Read the model definition and answer for the solid it produces. Units are mm, in the model's axes. Face numbers are marked on the shaded views. A direction names the side the tool comes from. Round coordinates to 2 decimals unless told otherwise and drop trailing zeros. Write each loop counter-clockwise with the first axis right and the second up, starting at its lowest first coordinate (ties: lowest second). Pieces come first, ordered by that corner, then holes. Notation, with made-up numbers: (-3, 42.25) - (5, 42.25) arc R25 cw to (5, 74.25) - close; hole circle Ø4 at (67.5, 42.25). An arc over 180 degrees is marked (long way). Answer as CSV lines item,"result". Start each with the question number.
1) For a pull along X with two mould halves and no side action, classify the marked faces 1, 2 and 3 as +X half, -X half, draft (parallel to the pull), parting line (faces both ways), or undercut.
2) Consider line 1 along Z through (x, y) = (12.7, 4.5); line 2 along X through (y, z) = (18.5, 19) (3 decimals); line 3 along Z through (x, y) = (-12.7, 2.25). Determine where each line is inside the solid, lowest interval first.
3) Find section D-D on y = 5.5. Determine the outline of the cut face in (x, z) (1 decimal), then the cut area to 3 significant figures.
4) Find section C-C on x = -12.7. Determine the outline of the cut face in (y, z).
5) Find section B-B on z = 34. Determine the outline of the cut face in (x, y) (3 decimals), then the cut area to 3 significant figures.
6) Which of the six approach directions +Z, -Z, +X, -X, +Y, -Y give full straight-line access (tool end or side, diameter ignored) to the marked faces 4, 5 and 6?
7) Find section A-A on y = 20.5. Determine the outline of the cut face in (x, z) (1 decimal), then the cut area to 3 significant figures.
8) Each of these flat-tipped pins is pushed along its axis until it touches: pin 1 (0.5 mm diameter, centred on x = 4, z = -0.5, fed in from +Y); pin 2 (4 mm diameter, centred on x = 12, y = 20, fed in from -Z); pin 3 (1 mm diameter, centred on x = 0, y = 9.5, fed in from +Z); pin 4 (8 mm diameter, centred on x = 4.5, y = 26.5, fed in from -Z). Where does it stop, or does it pass through?
Autodesk Inventor part; units mm, degrees
ref_plane "YZ Plane" through (0, 0, 0) normal (1, 0, 0) x (0, 1, 0)
ref_plane "XZ Plane" through (0, 0, 0) normal (0, 1, 0) x (-1, 0, 0)
ref_plane "XY Plane" through (0, 0, 0) normal (0, 0, 1) x (1, 0, 0)
sketch "Sketch1" plane through (0, 0, 0) normal (0, 0, 1) x (1, 0, 0)
  line L0 (-15.875, 0) -> (15.875, 0)
  line L1 (15.875, 0) -> (15.875, 38.1)
  line L2 (15.875, 38.1) -> (-15.875, 38.1)
  line L3 (-15.875, 38.1) -> (-15.875, 0)
  point P0 (0, 0)
  dimension "d2" = 31.75
  dimension "d3" = 38.1
  dimension "d4" = 15.875
  dimension "d5" = 0
extrude "Extrusion1" add sketch "Sketch1" along normal blind 139.7
sketch "Sketch2" plane through (0, 0, 139.7) normal (0, 0, 1) x (1, 0, 0)
  arc A0 (-12.065, 19.05) -> (12.065, 19.05) centre (0, 19.05) ccw
  line L0 (-15.875, 0) -> (15.875, 0)
  line L1 (12.065, 19.05) -> (12.065, 38.1)
  line L2 (15.875, 38.1) -> (-15.875, 38.1)
  line L3 (-12.065, 19.05) -> (-12.065, 38.1)
  point P0 (0, 0)
  dimension "d8" = 19.05
  dimension "d9" = 24.13
extrude "Extrusion2" cut sketch "Sketch2" against normal through all
sketch "Sketch3" plane through (-15.875, 0, 0) normal (0, -1, 0) x (1, 0, 0)
  circle A0 centre (28.575, 8.89) radius 2
  circle A1 centre (3.175, 130.81) radius 2
  line L0 (15.875, 0) -> (15.875, 139.7) construction
  line L1 (0, 139.7) -> (31.75, 139.7) construction
  line L2 (0, 0) -> (31.75, 0) construction
  line L3 (31.75, 139.7) -> (0, 139.7) construction
  circle A2 centre (3.175, 27.94) radius 2
  dimension "d12" = 4
  dimension "d13" = 4
  dimension "d14" = 12.7
  dimension "d15" = 8.89
  dimension "d16" = 12.7
  dimension "d17" = 8.89
  dimension "d28" = 4
  dimension "d30" = 12.7
  dimension "d31" = 27.94
extrude "Heat Set Inserts" cut sketch "Sketch3" against normal blind 7
sketch "Sketch4" plane through (0, 0, 139.7) normal (0, 0, 1) x (1, 0, 0)
  line L0 (-15.875, 0) -> (15.875, 0)
  line L1 (15.875, 0) -> (15.875, 38.1)
  line L2 (-15.875, 0) -> (15.875, 0)
  line L3 (15.875, 0) -> (15.875, 19.05)
  line L4 (15.875, 19.05) -> (-15.875, 19.05)
  line L5 (-15.875, 19.05) -> (-15.875, 0)
  point P0 (0, 0)
  dimension "d20" = 19.05
extrude "Back Wall" add sketch "Sketch4" along normal blind 1.5875
sketch "Sketch5" plane through (0, 0, 0) normal (0, 0, -1) x (-1, 0, 0)
  line L0 (15.875, 0) -> (-15.875, 0)
  line L1 (15.875, 19.05) -> (15.875, 0)
  line L2 (-15.875, 0) -> (15.875, 0)
  line L3 (15.875, 0) -> (15.875, 10.16)
  line L4 (15.875, 10.16) -> (-15.875, 10.16)
  line L5 (-15.875, 10.16) -> (-15.875, 0)
  point P0 (0, 0)
  dimension "d23" = 10.16
extrude "Extrusion5" add sketch "Sketch5" along normal blind 1.5875
sketch "Sketch6" plane through (0, 0, 141.2875) normal (0, 0, 1) x (1, 0, 0)
  line L0 (-12.065, 38.1) -> (-15.875, 38.1)
  line L1 (-15.875, 0) -> (15.875, 0)
  line L2 (-15.875, 38.1) -> (15.875, 38.1)
  line L3 (15.875, 38.1) -> (15.875, 0)
  line L4 (15.875, 0) -> (-15.875, 0)
  line L5 (-15.875, 0) -> (-15.875, 38.1)
  point P0 (0, 0)
extrude "Extrusion6" cut sketch "Sketch6" against normal blind 101.6
equation "\"d12\" = m3_heat_set_insert"
equation "\"d13\" = m3_heat_set_insert"
equation "\"d28\" = d29"
equation "\"d18\" = m3_heat_set_depth"
equation "\"m3_heat_set_insert\" = 4"
equation "\"m3_clearance\" = 3.4"
equation "\"m3_heat_set_depth\" = 7"
equation "\"robot_diameter\" = 354"
equation "\"hardboard_thickness\" = 5"
properties part number "NiMH_Holder_Front"
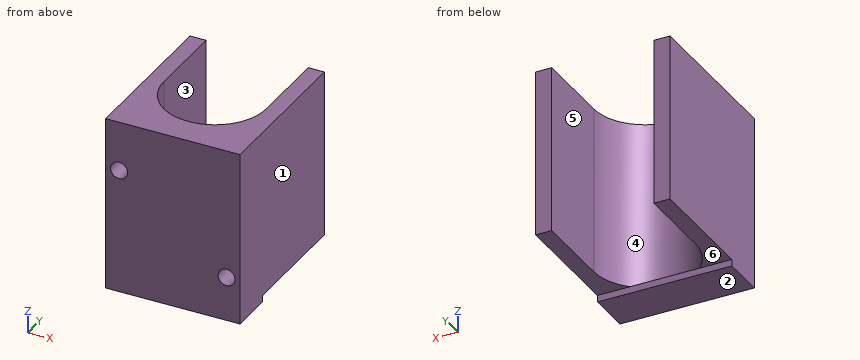
Check values:
1,face 1,"+X half"
1,face 2,"draft"
1,face 3,"undercut"
2,line 1,"z = -1.59 to 6.89, 10.89 to 39.69"
2,line 2,"x = -15.875 to -12.052, 12.052 to 15.875"
2,line 3,"z = -1.59 to 25.94, 29.94 to 39.69"
3,outline,"(-15.9, -1.6) - (15.9, -1.6) - (15.9, 39.7) - (-15.9, 39.7) - close; hole circle Ø4 at (-12.7, 27.9); hole circle Ø4 at (12.7, 8.9)"
3,area,"1,290 mm^2"
4,outline,"(0, -1.59) - (10.16, -1.59) - (10.16, 0) - (38.1, 0) - (38.1, 39.69) - (0, 39.69) - (0, 29.94) - (7, 29.94) - (7, 25.94) - (0, 25.94) - close"
5,outline,"(-15.875, 0) - (15.875, 0) - (15.875, 38.1) - (12.065, 38.1) - (12.065, 19.05) arc R12.065 cw to (-12.065, 19.05) - (-12.065, 38.1) - (-15.875, 38.1) - close"
5,area,"521 mm^2"
6,face 4,"+Z, +Y"
6,face 5,"+Z, -Z, +Y"
6,face 6,"-Z, +X, -X, +Y"
7,outline,"(-15.9, 0) - (-12.1, 0) - (-12.1, 39.7) - (-15.9, 39.7) - close; (12.1, 0) - (15.9, 0) - (15.9, 39.7) - (12.1, 39.7) - close"
7,area,"302 mm^2"
8,pin 1,"stops at y = 10.16"
8,pin 2,"stops at z = 0"
8,pin 3,"stops at z = 0"
8,pin 4,"passes through"
